Check sheet for the modelled part. Datum: model origin and axes. Units: mm. A direction names the side the tool comes from. Round coordinates to 2 decimals unless told otherwise and drop trailing zeros. Write each loop counter-clockwise with the first axis right and the second up, starting at its lowest first coordinate (ties: lowest second). Pieces come first, ordered by that corner, then holes. Notation, with made-up numbers: (28.5, 25) -> (33.5, 25) arc R16 cw to (33.5, 44) -> close; hole circle Ø3 at (33.25, 29.5). An arc over 180 degrees is marked (long way). Put each result on its own line as item: value. Start each with the question number.
from build123d import *

# Parameters (mm, degrees)
F1_R     = 12
F1_R_2   = 6
F2_DEPTH = 40
F1_R_3   = 2.25
F3_DEPTH = 10
F4_R     = 2.5
F5_R     = 0.5


with BuildPart() as f2:
    # F1 (on Front) → F2 (new body)
    with BuildSketch(Plane.XZ):
        Circle(F1_R)
        Circle(F1_R_2, mode=Mode.SUBTRACT)
    extrude(amount=-F2_DEPTH)

    # F1 (on Front) → F3 (join)
    with BuildSketch(Plane.XZ):
        with BuildLine():
            Line((13.228757, 15), (-13.228757, 15))
            ThreePointArc((-13.228757, 15), (-20, 0), (-13.228757, -15))
            Line((-13.228757, -15), (13.228757, -15))
            ThreePointArc((13.228757, -15), (20, 0), (13.228757, 15))
        make_face()
        with Locations((-11.313708, -11.313708)):
            Circle(F1_R_3, mode=Mode.SUBTRACT)
        with Locations((-16, 0)):
            Circle(F1_R_3, mode=Mode.SUBTRACT)
        Circle(F1_R, mode=Mode.SUBTRACT)
        with Locations((11.313708, -11.313708)):
            Circle(F1_R_3, mode=Mode.SUBTRACT)
        with Locations((16, 0)):
            Circle(F1_R_3, mode=Mode.SUBTRACT)
        with Locations((-11.313708, 11.313708)):
            Circle(F1_R_3, mode=Mode.SUBTRACT)
        with Locations((11.313708, 11.313708)):
            Circle(F1_R_3, mode=Mode.SUBTRACT)
    extrude(amount=-F3_DEPTH)

    # F4
    f4_edges = [f2.edges().sort_by_distance(p)[0] for p in [
        (-13.228757, 5, 15),
        (-13.228757, 5, -15),
        (13.228757, 5, 15),
        (13.228757, 5, -15),
    ]]
    fillet(f4_edges, radius=F4_R)

    # F5
    f5_edges = [f2.edges().sort_by_distance(p)[0] for p in [
        (20, 10, 0),
        (20, 0, 0),
        (-12, 10, 0),
        (-12, 40, 0),
    ]]
    fillet(f5_edges, radius=F5_R)


solid = f2.part
1. Access from +Z, -Z, +X, -X, +Y, -Y to the whole of each face (thin tool, end or side, straight path). Record for faces 1 (the flat face through (0, 5, 15)), 2 (the cylindrical face through (-11.99, 24.8, 0.53)).
2. Section check D-D, the plane y = 25. Enter the section's corners in (x, z).
3. Gauge pin test, flat ends, axial feed: P1, Ø5, axis at x = 11.31, z = 11.31, coming from the +Y side; P2, Ø2.5, axis at x = -11.31, z = 11.31, coming from the +Y side; P3, Ø12, axis at y = 28, z = -5, coming from the +X side; P4, Ø5, axis at x = 8.5, y = 25, coming from the +Z side. Record the tip position at first contact, or that the pin passes through.
4. Section check B-B, the plane z = 0. Enter the section's corners in (x, y).
5. Section check C-C, the plane y = 5. Enter the section's corners in (x, z), then the cut area to 3 significant figures.
6. Section check A-A, the plane x = 0. Enter the section's corners in (y, z).
7. Material ranges on L1, parallel to Z at x = 10.5, y = 2; L2, parallel to Z at x = 16, y = 6.5; L3, parallel to X at y = 9, z = -1.25, recorded low to high. Write a range as [from, to].
Reply:
1. face 1: +Z, +X, -X, +Y, -Y
1. face 2: +Y
2. outline: circle Ø24 at (0, 0); hole circle Ø12 at (0, 0)
3. P1: stops at y = 10
3. P2: passes through
3. P3: stops at x = 12
3. P4: stops at z = 10.39
4. outline: (-20, 0.5) arc R0.5 ccw to (-19.5, 0) -> (-18.25, 0) -> (-18.25, 10) -> (-19.5, 10) arc R0.5 ccw to (-20, 9.5) -> close; (-13.75, 0) -> (-6, 0) -> (-6, 40) -> (-11.5, 40) arc R0.5 ccw to (-12, 39.5) -> (-12, 10.5) arc R0.5 cw to (-12.5, 10) -> (-13.75, 10) -> close; (6, 0) -> (13.75, 0) -> (13.75, 10) -> (12.5, 10) arc R0.5 cw to (12, 10.5) -> (12, 39.5) arc R0.5 ccw to (11.5, 40) -> (6, 40) -> close; (18.25, 0) -> (19.5, 0) arc R0.5 ccw to (20, 0.5) -> (20, 9.5) arc R0.5 ccw to (19.5, 10) -> (18.25, 10) -> close
5. outline: (-14, -14.29) arc R2.5 ccw to (-12.25, -15) -> (12.25, -15) arc R2.5 ccw to (14, -14.29) arc R20 ccw to (14, 14.29) arc R2.5 ccw to (12.25, 15) -> (-12.25, 15) arc R2.5 ccw to (-14, 14.29) arc R20 ccw to start; hole circle Ø4.5 at (-16, 0); hole circle Ø4.5 at (-11.31, -11.31); hole circle Ø4.5 at (-11.31, 11.31); hole circle Ø12 at (0, 0); hole circle Ø4.5 at (11.31, -11.31); hole circle Ø4.5 at (11.31, 11.31); hole circle Ø4.5 at (16, 0)
5. area: 866 mm2
6. outline: (0, -14.5) arc R0.5 ccw to (0.5, -15) -> (9.5, -15) arc R0.5 ccw to (10, -14.5) -> (10, -12.5) arc R0.5 cw to (10.5, -12) -> (39.5, -12) arc R0.5 ccw to (40, -11.5) -> (40, -6) -> (0, -6) -> close; (0, 6) -> (40, 6) -> (40, 11.5) arc R0.5 ccw to (39.5, 12) -> (10.5, 12) arc R0.5 cw to (10, 12.5) -> (10, 14.5) arc R0.5 ccw to (9.5, 15) -> (0.5, 15) arc R0.5 ccw to (0, 14.5) -> close
7. L1: z = [-15, -13.41], [-9.22, 9.22], [13.41, 15]
7. L2: z = [-12, -2.25], [2.25, 12]
7. L3: x = [-19.96, -17.87], [-14.13, -5.87], [5.87, 14.13], [17.87, 19.96]
